The listing builds one solid part. Answer for the finished solid, in the listing's coordinates (mm). A direction names the side the tool comes from. Round coordinates to 2 decimals unless told otherwise and drop trailing zeros. Write each loop counter-clockwise with the first axis right and the second up, starting at its lowest first coordinate (ties: lowest second). Pieces come first, ordered by that corner, then holes. Notation, with made-up numbers: M 25,77.25 L 66,77.25 A18 cw 66,98.25 Z; hole C 17.5,-37.5 d3. An arc over 180 degrees is marked long. One line per item, written item: value. Start each with the question number.
(1) Consider probe 1 along Z at (x, y) = (6.06, 1.4); probe 2 along Z at (x, y) = (10, 8); probe 3 along Z at (x, y) = (-12, -2.75). Determine where each line is inside the solid, lowest interval first.
(2) For a pull along Z with two mould halves and no side action, classify faces 1 (the flat face through (9, -4, 88.05)), 2 (the cylindrical face through (-17.88, 8.57, 34.53)), 3 (the flat face through (14, 0, 26.8)) as released by +Z, released by -Z, zero draft, split by the parting line, or undercut.
(3) For faces 4 (the flat face through (6, 6, 46)), 5 (the flat face through (-4.98, 0, -2)), 6 (the flat face through (16.62, 0, 67)), 7 (the flat face through (6, -3, 95)), determine the directions among +Z, -Z, +X, -X, +Y, -Y from which every point of the face is accessible in a straight line to the end or side of a thin tool.
(4) Section D-D (x = -6) is taken. Determine the outline of the cut face in (y, z), plus the area to 3 significant figures.
(5) Given P1, Ø8, axis at y = -6, z = 76.5, coming from the -X side; P2, Ø9.5, axis at x = 5.5, z = 37.5, coming from the +Y side; P3, Ø9.5, axis at y = -2.5, z = 82.5, coming from the +X side, each flat-ended and moving along its own axis, determine where each tip first touches the part or whether it passes through.
(6) Section B-B (z = 33) is taken. Determine the outline of the cut face in (x, y), plus the area to 3 significant figures.
(7) Section A-A (z = 92.55) is taken. Determine the outline of the cut face in (x, y).
(8) Section C-C (y = 7.5) is taken. Determine the outline of the cut face in (x, z).
```python
from build123d import *

# Parameters (mm, degrees)
F1_DEPTH  = 10
F0_R      = 2.09
F2_DEPTH  = 4
F3_DEPTH  = 6
F0_W      = 12.12
F0_H      = 38
F4_DEPTH  = 6
F6_R      = 0.5
F7_DEPTH  = 36
F8_R      = 5
F10_R     = 4.45
F11_DEPTH = 1.5
F0_R_2    = 2
F12_DEPTH = 3
F13_DEPTH = 25
F14_R     = 0.5


with BuildPart() as f1:
    # F0 (on Front) → F1 (new body, symmetric)
    with BuildSketch(Plane.XZ):
        Polygon((-19.38, 0), (-4.98, 0), (0, 0), (4.98, 0), (16.62, 0), (16.62, 26.8), (12.12, 26.8), (0, 26.8), (0, 64.8), (12.12, 64.8), (16.62, 64.8), (16.62, 70.05), (12.12, 70.05), (0, 70.05), (-3, 70.05), (-19.38, 70.05), align=None)
    extrude(amount=F1_DEPTH, both=True)

    # F0 (on Front) → F2 (join, symmetric)
    with BuildSketch(Plane.XZ):
        with BuildLine():
            Line((0, 0), (-4.98, 0))
            Line((-4.98, 0), (-4.98, -4.62))
            ThreePointArc((-4.98, -4.62), (-3.7557063454, -7.5757063454), (-0.8, -8.8))
            Line((-0.8, -8.8), (0.8, -8.8))
            ThreePointArc((0.8, -8.8), (3.7557063454, -7.5757063454), (4.98, -4.62))
            Line((4.98, -4.62), (4.98, 0))
            Line((4.98, 0), (0, 0))
        make_face()
        with Locations((0, -4.4)):
            Circle(F0_R, mode=Mode.SUBTRACT)
    extrude(amount=F2_DEPTH, both=True)

    # F0 (on Front) → F3 (join, symmetric)
    with BuildSketch(Plane.XZ):
        Polygon((0, 88.05), (0, 70.05), (12.12, 70.05), (12.12, 88.05), (10.56, 88.05), (1.56, 88.05), align=None)
    extrude(amount=F3_DEPTH, both=True)

    # F0 (on Front) → F4 (join, symmetric)
    with BuildSketch(Plane.XZ):
        with Locations((6.06, 45.8)):
            Rectangle(F0_W, F0_H)
    extrude(amount=F4_DEPTH, both=True)

    # F6 (on plane+point) → F7 (join)
    with BuildSketch(Plane.XY.offset(70.05)):
        with Locations((-3, 0)):
            Circle(F6_R)
    extrude(amount=F7_DEPTH)

    # F8
    f8_edges = [f1.edges().sort_by_distance(p)[0] for p in [
        (-19.38, 10, 35.025),
        (-19.38, -10, 35.025),
        (16.62, 10, 13.4),
        (16.62, -10, 13.4),
        (16.62, 10, 67.425),
        (16.62, -10, 67.425),
    ]]
    fillet(f8_edges, radius=F8_R)

    # F10 (on offset) → F11 (join)
    with BuildSketch(Plane.XY.offset(88.05)):
        with Locations((6.06, 0)):
            Circle(F10_R)
    extrude(amount=F11_DEPTH)

    # F0 (on Front) → F12 (join, symmetric)
    with BuildSketch(Plane.XZ):
        with BuildLine():
            Line((1.56, 93.05), (1.56, 89.55))
            Line((1.56, 89.55), (10.56, 89.55))
            Line((10.56, 89.55), (10.56, 93.05))
            ThreePointArc((10.56, 93.05), (9.3884271247, 95.8784271247), (6.56, 97.05))
            Line((6.56, 97.05), (5.56, 97.05))
            ThreePointArc((5.56, 97.05), (2.7315728753, 95.8784271247), (1.56, 93.05))
        make_face()
        with Locations((6.06, 92.55)):
            Circle(F0_R_2, mode=Mode.SUBTRACT)
    extrude(amount=F12_DEPTH, both=True)

    # F13 (cut): a face of the model
    f13_faces = [f1.faces().sort_by_distance(p)[0] for p in [
        (0.1705562664, 0, 88.05),
    ]]
    extrude(f13_faces, amount=F13_DEPTH, mode=Mode.SUBTRACT)

    # F14
    f14_edges = [f1.edges().sort_by_distance(p)[0] for p in [
        (4.98, -4, -2.31),
        (4.98, 4, -2.31),
        (-4.98, -4, -2.31),
        (-4.98, 4, -2.31),
    ]]
    fillet(f14_edges, radius=F14_R)


solid = f1.part
```
Recorded:
1. probe 1: z = 0 to 90.55, 94.55 to 97.05
1. probe 2: z = 0 to 26.8, 64.8 to 70.05
1. probe 3: z = 0 to 70.05
2. face 1: released by +Z
2. face 2: zero draft
2. face 3: undercut
3. face 4: +X, +Y
3. face 5: -Z, -X, +Y, -Y
3. face 6: +Z, -Z, +X, +Y, -Y
3. face 7: +Z, +X, -X, -Y
4. outline: M -10,0 L 10,0 L 10,70.05 L -10,70.05 Z
4. area: 1,400 mm2
5. P1: stops at x = 0
5. P2: stops at y = 6
5. P3: stops at x = 12.12
6. outline: M -19.38,-5 A5 ccw -14.38,-10 L 0,-10 L 0,-6 L 12.12,-6 L 12.12,6 L 0,6 L 0,10 L -14.38,10 A5 ccw -19.38,5 Z
6. area: 522 mm2
7. outline: C -3,0 d1; M 2.77,-3 L 4.06,-3 L 4.06,3 L 2.77,3 A4.45 ccw Z; M 8.06,-3 L 9.35,-3 A4.45 ccw 9.35,3 L 8.06,3 Z
8. outline: M -18.71,0 L 15.95,0 L 15.95,26.8 L 0,26.8 L 0,64.8 L 15.95,64.8 L 15.95,70.05 L -18.71,70.05 Z
